```python
from build123d import *

# Parameters (mm, degrees)
SKETCH1_W            = 11.9
SKETCH1_H            = 5.08
SKETCH1_H_2          = 16.5
SKETCH1_H_3          = 0.635
BOSS_EXTRUDE1_DEPTH  = 1.27
SKETCH1_3_W          = 11.9
SKETCH1_3_H          = 5.08
BOSS_EXTRUDE2_DEPTH  = 16.77
SKETCH2_R            = 1.1
CUT_EXTRUDE1_DEPTH   = 10.16
SKETCH3_R            = 1.1
CUT_EXTRUDE2_DEPTH   = 10.16
SKETCH4_W            = 22.85
SKETCH4_H            = 1.48
SKETCH4_W_2          = 5.08
BOSS_EXTRUDE4_DEPTH  = 11.9
SKETCH6_W            = 22.85
SKETCH6_H            = 2.75
SKETCH6_W_2          = 5.08
BOSS_EXTRUDE5_DEPTH  = 11.9
SKETCH7_W            = 5.08
SKETCH7_H            = 1.375
SKETCH7_W_2          = 22.85
BOSS_EXTRUDE6_DEPTH  = 2.5
BOSS_EXTRUDE7_DEPTH  = 2.5
BOSS_EXTRUDE13_START = 0.5
SKETCH19_W           = 11.9
SKETCH19_H           = 5.08
SKETCH19_R           = 1.1
BOSS_EXTRUDE13_DEPTH = 0.5
BOSS_EXTRUDE14_DEPTH = 24.7
SKETCH21_W           = 24.7
SKETCH21_H           = 27.93
BOSS_EXTRUDE16_DEPTH = 0.5
SKETCH23_W           = 12.35
SKETCH23_H           = 3.33
SKETCH23_H_2         = 1.75
BOSS_EXTRUDE17_DEPTH = 15.5
SKETCH24_R           = 1.1
CUT_EXTRUDE3_DEPTH   = 10


with BuildPart() as part:
    # Sketch1 → Boss-Extrude1 (new body)
    with BuildSketch(Plane(origin=(0, 0, 0), x_dir=(1, 0, 0), z_dir=(0, 1, 0))):
        with Locations((5.95, 19.675)):
            Rectangle(SKETCH1_W, SKETCH1_H)
        with Locations((5.95, 8.25)):
            Rectangle(SKETCH1_W, SKETCH1_H_2)
        with Locations((5.95, 16.8175)):
            Rectangle(SKETCH1_W, SKETCH1_H_3)
        with Locations((5.95, -3.175)):
            Rectangle(SKETCH1_W, SKETCH1_H)
        with Locations((5.95, -0.3175)):
            Rectangle(SKETCH1_W, SKETCH1_H_3)
    extrude(amount=BOSS_EXTRUDE1_DEPTH)

    # Sketch1_3 → Boss-Extrude2 (add)
    with BuildSketch(Plane(origin=(0, 0, 0), x_dir=(1, 0, 0), z_dir=(0, 1, 0))):
        with Locations((5.95, -3.175)):
            Rectangle(SKETCH1_3_W, SKETCH1_3_H)
        with Locations((5.95, 19.675)):
            Rectangle(SKETCH1_3_W, SKETCH1_3_H)
    extrude(amount=BOSS_EXTRUDE2_DEPTH)

    # Sketch2 → Cut-Extrude1 (cut)
    with BuildSketch(Plane(origin=(0, 16.77, 0), x_dir=(1, 0, 0), z_dir=(0, 1, 0))):
        with Locations(Location((5.95, 19.765430595, 0), (0, 0, 270))):
            Circle(SKETCH2_R)
    extrude(amount=-CUT_EXTRUDE1_DEPTH, mode=Mode.SUBTRACT)

    # Sketch3 → Cut-Extrude2 (cut)
    with BuildSketch(Plane(origin=(0, 16.77, 0), x_dir=(1, 0, 0), z_dir=(0, 1, 0))):
        with Locations(Location((5.95, -3.056330688, 0), (0, 0, 270))):
            Circle(SKETCH3_R)
    extrude(amount=-CUT_EXTRUDE2_DEPTH, mode=Mode.SUBTRACT)

    # Sketch4 → Boss-Extrude4 (add)
    with BuildSketch(Plane(origin=(11.9, 0, 0), x_dir=(0, 0, -1), z_dir=(1, 0, 0))):
        with Locations((10.79, -0.74)):
            Rectangle(SKETCH4_W, SKETCH4_H)
        with Locations((-3.175, -0.74)):
            Rectangle(SKETCH4_W_2, SKETCH4_H)
    extrude(amount=-BOSS_EXTRUDE4_DEPTH)

    # Sketch6 → Boss-Extrude5 (add)
    with BuildSketch(Plane(origin=(11.9, 0, 0), x_dir=(0, 0, -1), z_dir=(1, 0, 0))):
        with Locations((10.79, -2.855)):
            Rectangle(SKETCH6_W, SKETCH6_H)
        with Locations((-3.175, -2.855)):
            Rectangle(SKETCH6_W_2, SKETCH6_H)
    extrude(amount=-BOSS_EXTRUDE5_DEPTH)

    # Sketch7 → Boss-Extrude6 (add)
    with BuildSketch(Plane(origin=(11.9, 0, 0), x_dir=(0, 0, -1), z_dir=(1, 0, 0))):
        with Locations((-3.175, -3.5425)):
            Rectangle(SKETCH7_W, SKETCH7_H)
        with Locations((-3.175, -4.9175)):
            Rectangle(SKETCH7_W, SKETCH7_H)
        with Locations((10.79, -3.5425)):
            Rectangle(SKETCH7_W_2, SKETCH7_H)
        with Locations((10.79, -4.9175)):
            Rectangle(SKETCH7_W_2, SKETCH7_H)
    extrude(amount=BOSS_EXTRUDE6_DEPTH)

    # Sketch8 → Boss-Extrude7 (add)
    with BuildSketch(Plane(origin=(11.9, 0, 0), x_dir=(0, 0, -1), z_dir=(1, 0, 0))):
        Polygon((22.215, -1.63), (-0.635, -1.63), (-5.715, -1.63), (-5.715, -2.855), (22.215, -2.855), align=None)
    extrude(amount=BOSS_EXTRUDE7_DEPTH)

    # Sketch19 → Boss-Extrude13 (add)
    # profile 1 of 2: a face of its own
    with BuildSketch(Plane(origin=(0, 16.77, 0), x_dir=(1, 0, 0), z_dir=(0, 1, 0)).offset(BOSS_EXTRUDE13_START)):
        with Locations((5.95, 19.675)):
            Rectangle(SKETCH19_W, SKETCH19_H)
        with Locations(Location((5.95, 19.765430595, 0), (0, 0, 270))):
            Circle(SKETCH19_R, mode=Mode.SUBTRACT)
    # profile 2 of 2: a face of its own
    with BuildSketch(Plane(origin=(0, 16.77, 0), x_dir=(1, 0, 0), z_dir=(0, 1, 0)).offset(BOSS_EXTRUDE13_START)):
        with Locations((5.95, -3.175)):
            Rectangle(SKETCH19_W, SKETCH19_H)
        with Locations(Location((5.95, -3.056330688, 0), (0, 0, 270))):
            Circle(SKETCH19_R, mode=Mode.SUBTRACT)
    extrude(amount=-BOSS_EXTRUDE13_DEPTH)

    # Sketch20 → Boss-Extrude14 (add)
    with BuildSketch(Plane(origin=(14.4, 0, 0), x_dir=(0, 0, -1), z_dir=(1, 0, 0))):
        Polygon((-5.715, -1.63), (-5.715, -4.38), (22.215, -4.38), (22.215, -3.6175), (22.215, 1.27), (-5.715, 1.27), align=None)
    extrude(amount=BOSS_EXTRUDE14_DEPTH)

    # Sketch21 → Boss-Extrude16 (add)
    with BuildSketch(Plane(origin=(0, 1.27, 0), x_dir=(1, 0, 0), z_dir=(0, 1, 0))):
        with Locations((26.75, 8.25)):
            Rectangle(SKETCH21_W, SKETCH21_H)
    extrude(amount=BOSS_EXTRUDE16_DEPTH)

    # Sketch23 → Boss-Extrude17 (add)
    with BuildSketch(Plane(origin=(0, 1.77, 0), x_dir=(1, 0, 0), z_dir=(0, 1, 0))):
        with Locations((20.575, 20.55)):
            Rectangle(SKETCH23_W, SKETCH23_H)
        with Locations((20.575, 23.09)):
            Rectangle(SKETCH23_W, SKETCH23_H_2)
        with Locations((32.925, 23.09)):
            Rectangle(SKETCH23_W, SKETCH23_H_2)
        with Locations((32.925, 20.55)):
            Rectangle(SKETCH23_W, SKETCH23_H)
        with Locations((32.925, -4.05)):
            Rectangle(SKETCH23_W, SKETCH23_H)
        with Locations((32.925, -6.59)):
            Rectangle(SKETCH23_W, SKETCH23_H_2)
        with Locations((20.575, -4.05)):
            Rectangle(SKETCH23_W, SKETCH23_H)
        with Locations((20.575, -6.59)):
            Rectangle(SKETCH23_W, SKETCH23_H_2)
    extrude(amount=BOSS_EXTRUDE17_DEPTH)

    # Sketch24 → Cut-Extrude3 (cut)
    with BuildSketch(Plane(origin=(0, 17.27, 0), x_dir=(1, 0, 0), z_dir=(0, 1, 0))):
        with Locations(Location((26.75, 20.675, 0), (0, 0, 270))):
            Circle(SKETCH24_R)
        with Locations(Location((26.75, -4.069787702, 0), (0, 0, 270))):
            Circle(SKETCH24_R)
    extrude(amount=-CUT_EXTRUDE3_DEPTH, mode=Mode.SUBTRACT)


solid = part.part
```
Can you work these out from the model? Positions are in its coordinate system, mm. A direction names the side the tool comes from. Round coordinates to 2 decimals unless told otherwise and drop trailing zeros. Order: outer loops, then holes, each group sorted by start corner. A loop starts at its lowest first (then second) coordinate and runs counter-clockwise, first axis right, second up. Notation, with made-up numbers: (21.25, 2.5) -> (43.25, 2.5) arc R22 ccw to (43.25, 23.5) -> close; hole circle Ø3 at (-21, 38.5). An arc over 180 degrees is marked (long way). Return JSON: item names as keys, results as strings. Group by question number.
1. If we section it at B-B, the plane y = 0: Write out the boundary of the cut face in (x, z) (3 decimals).
2. Which directions (+Z, -Z, +X, -X, +Y, -Y) give clear straight access to the entire face, cutting with the end or side of a thin tool? Please do faces 5 (the face through (11.9, 0, -8)), 6 (the face through (27, 7.27, -21)), 7 (the face through (11, 6, 5.715)), 8 (the face through (6, -4.23, -8)).
3. Will these pins go through, and if not, where does the flat tip stop? pin 1 (6 mm diameter, centred on x = 8, y = 8.5, fed in from -Z) (3 decimals); pin 2 (2.5 mm diameter, centred on x = 5.95, z = 3.06, fed in from -Y); pin 3 (1.4 mm diameter, centred on x = 22.5, z = 6.5, fed in from -Y).
4. I need wall thicknesses on line 1 (X direction, y = 0, z = -7); line 2 (Z direction, x = 34, y = 5.75) (3 decimals); line 3 (X direction, y = 7.75, z = -19.5). Which ranges of each line are inside material? Lowest first, please. Write a range as [from, to].
5. If we section it at D-D, the plane x = 7.5: Write out the boundary of the cut face in (y, z) (3 decimals).
6. If we section it at A-A, the plane y = 11.75: Write out the boundary of the cut face in (x, z) (3 decimals), then the cut area to 3 significant figures.
7. We'd pull the mould along X, two halves only. Please class faces 1 (the face through (27, 7.27, 4)), 2 (the face through (6.693, 12.015, 2.246)), 3 (the face through (0, 0, -8)), 4 (the face through (6, 9, -17.135)): released by +X, released by -X, zero draft, split by the parting line, or undercut.
8. If we section it at C-C, the plane z = -1.5: Write out the boundary of the cut face in (x, y) (3 decimals).
Output values:
{
 "1": {"outline": "(0, -22.215) -> (11.9, -22.215) -> (11.9, 5.715) -> (0, 5.715) -> close; (14.4, -22.215) -> (39.1, -22.215) -> (39.1, 5.715) -> (14.4, 5.715) -> close"},
 "2": {"face 5": "+Z, -Z, +Y", "face 6": "+Y", "face 7": "+Z, -X, -Y", "face 8": "+Z, -Z, -X, -Y"},
 "3": {"pin 1": "z = -22.215", "pin 2": "y = -4.23", "pin 3": "y = 1.77"},
 "4": {"line 1": "[0, 11.9], [14.4, 39.1]", "line 2": "[-23.965, -18.885], [2.385, 7.465]", "line 3": "[0, 4.88], [7.02, 11.9], [14.4, 39.1]"},
 "5": {"outline": "(-4.23, -22.215) -> (17.27, -22.215) -> (17.27, -17.135) -> (1.27, -17.135) -> (1.27, 0.635) -> (17.27, 0.635) -> (17.27, 5.715) -> (-4.23, 5.715) -> close"},
 "6": {"outline": "(0, -22.215) -> (11.9, -22.215) -> (11.9, -17.135) -> (0, -17.135) -> close; (0, 0.635) -> (11.9, 0.635) -> (11.9, 5.715) -> (0, 5.715) -> close; (14.4, -23.965) -> (39.1, -23.965) -> (39.1, -18.885) -> (14.4, -18.885) -> close; (14.4, 2.385) -> (39.1, 2.385) -> (39.1, 7.465) -> (14.4, 7.465) -> close; hole circle Ø2.2 at (5.95, -19.765); hole circle Ø2.2 at (5.95, 3.056); hole circle Ø2.2 at (26.75, -20.675); hole circle Ø2.2 at (26.75, 4.07)", "area": "357 mm²"},
 "7": {"face 1": "undercut", "face 2": "undercut", "face 3": "released by -X", "face 4": "zero draft"},
 "8": {"outline": "(0, -4.23) -> (11.9, -4.23) -> (11.9, -5.605) -> (14.4, -5.605) -> (14.4, -4.38) -> (39.1, -4.38) -> (39.1, 1.77) -> (14.4, 1.77) -> (14.4, -1.63) -> (11.9, -1.63) -> (11.9, 1.27) -> (0, 1.27) -> close"}
}
